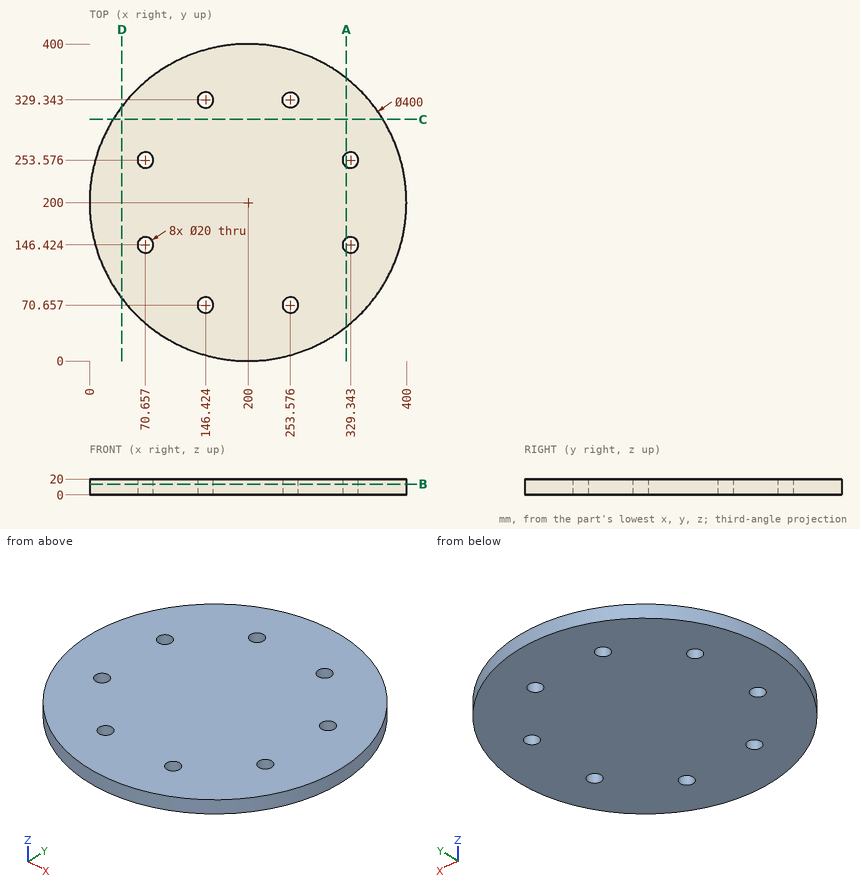
Job drawing, mm, ordinate dimensions from the low corner. One solid piece. Give positions to 0.01 mm unless a question says otherwise; leave off trailing zeros. Loops run counter-clockwise (first coordinate to the right, second up) from the corner with the lowest first, then second, coordinate; pieces in that order, holes last.
Item 1: Slice it at A-A, the plane x = 324. List the corners of the cut face in (y, z), and give its area (3 significant figures).
Answers follow:
outline: (43.08, 0) - (137.97, 0) - (137.97, 20) - (43.08, 20) - close; (154.88, 0) - (245.12, 0) - (245.12, 20) - (154.88, 20) - close; (262.03, 0) - (356.92, 0) - (356.92, 20) - (262.03, 20) - close
area: 5,600 mm2
Item 2: Slice it at B-B, the plane z = 13.5. Give the number of separate pieces and of enclosed holes in the cut face, and give its area (3 significant figures).
Answers follow:
separate pieces: 1
enclosed holes: 8
area: 123,000 mm2
Item 3: Drill centre lines: line 1 (X direction, y = 325.5, z = 15.25) (1 decimal); line 2 (Y direction, x = 251.5, z = 16.75) (1 decimal); line 3 (Y direction, x = 258.5, z = 7). Where is each one in solid material? Low to high.
Answers follow:
line 1: x = 44.3 to 137.2, 155.7 to 244.3, 262.8 to 355.7
line 2: y = 6.7 to 60.9, 80.4 to 319.6, 339.1 to 393.3
line 3: y = 8.75 to 61.95, 79.36 to 320.64, 338.05 to 391.25
Item 4: Flat gauge pins, fed straight in: pin 1 (2 mm diameter, centred on y = 213, z = 9.5, fed in from +X); pin 2 (3 mm diameter, centred on y = 290.5, z = 11, fed in from -X); pin 3 (5 mm diameter, centred on x = 187, z = 11, fed in from +Y). Where does each tip first touch, or does it go through?
Answers follow:
pin 1: stops at x = 399.64
pin 2: stops at x = 20.89
pin 3: stops at y = 399.72
Item 5: Slice it at C-C, the plane y = 305. List the corners of the cut face in (x, z), and give its area (3 significant figures).
Answers follow:
outline: (29.78, 0) - (370.22, 0) - (370.22, 20) - (29.78, 20) - close
area: 6,810 mm2
Item 6: Slice it at D-D, the plane x = 41. List the corners of the cut face in (y, z).
Answers follow:
outline: (78.68, 0) - (321.32, 0) - (321.32, 20) - (78.68, 20) - close
